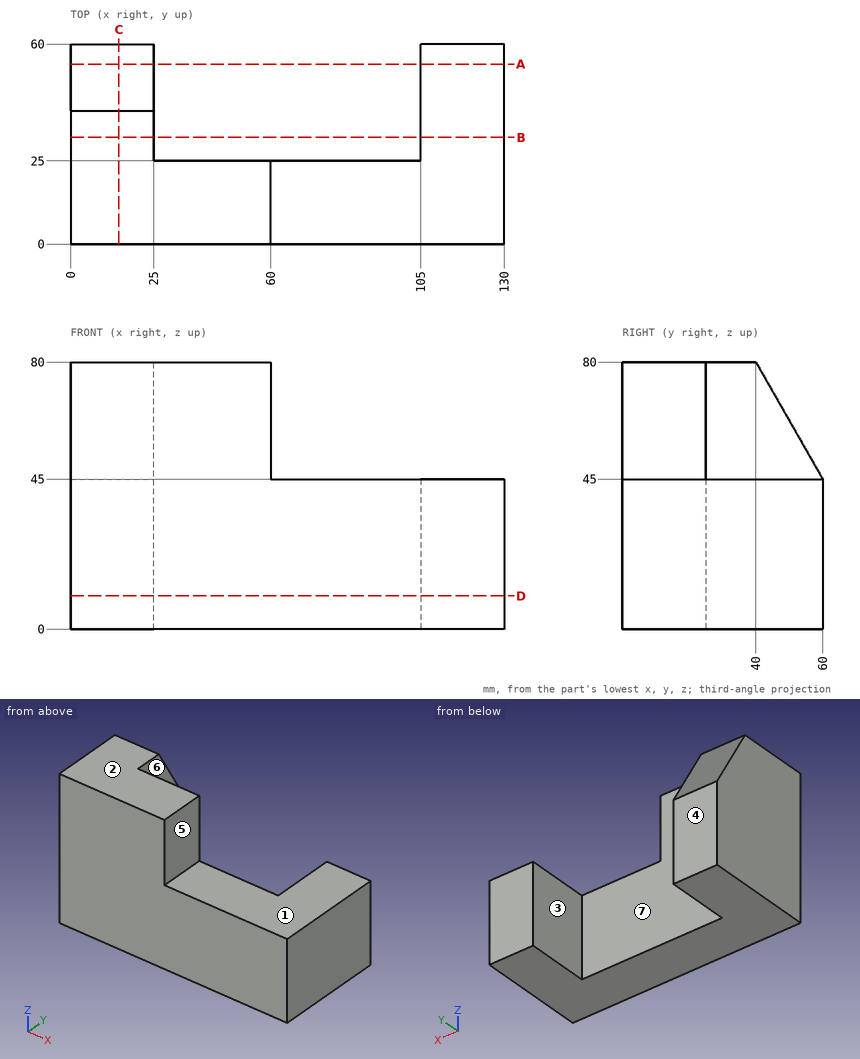
Could you check a few things on this drawing? It's one solid part, dimensions in mm from its lowest x, y, z. A direction names the side the tool comes from. Round coordinates to 2 decimals unless told otherwise and drop trailing zeros. Order: outer loops, then holes, each group sorted by start corner. A loop starts at its lowest first (then second) coordinate and runs counter-clockwise, first axis right, second up. Notation, with made-up numbers: M -3.75,-9.5 L 32.25,-9.5 A15 ccw 32.25,6.5 Z; hole C 47.25,52.5 d3. An arc over 180 degrees is marked long. Use a Markdown table: item, result.
1) Imagine slicing it at B-B (y = 32). List the corners of the cut face in (x, z) for me, then the cut area to 4 significant figures.
Geometry says:
| item | result |
|---|---|
| outline | M 0,0 L 25,0 L 25,80 L 0,80 Z; M 105,0 L 130,0 L 130,45 L 105,45 Z |
| area | 3,125 mm² |
2) I'm going to push flat-ended pins straight in: P1, Ø10.5, axis at y = 51, z = 12.5, coming from the -X side; P2, Ø5, axis at x = 69, z = 40, coming from the +Y side. Where does each tip first touch, or does it pass through?
Geometry says:
| item | result |
|---|---|
| P1 | stops at x = 0 |
| P2 | stops at y = 25 |
3) Imagine slicing it at A-A (y = 54). List the corners of the cut face in (x, z) for me.
Geometry says:
| item | result |
|---|---|
| outline | M 0,0 L 25,0 L 25,55.5 L 0,55.5 Z; M 105,0 L 130,0 L 130,45 L 105,45 Z |
4) Imagine slicing it at D-D (z = 10). List the corners of the cut face in (x, y) for me.
Geometry says:
| item | result |
|---|---|
| outline | M 0,0 L 130,0 L 130,60 L 105,60 L 105,25 L 25,25 L 25,60 L 0,60 Z |
5) Imagine slicing it at C-C (x = 14.5). List the corners of the cut face in (y, z) for me, then the cut area to 3 significant figures.
Geometry says:
| item | result |
|---|---|
| outline | M 0,0 L 60,0 L 60,45 L 40,80 L 0,80 Z |
| area | 4,450 mm² |
6) On a 3-axis mill with a long thin cutter (end or side, diameter ignored), from which of +Z, -Z, +X, -X, +Y, -Y can I reach the whole of each face in a straight line? I mean the marked faces 1, 2 and 3. Say none if no direction works.
Geometry says:
| item | result |
|---|---|
| face 1 | +Z, +X, +Y, -Y |
| face 2 | +Z, +X, -X, +Y, -Y |
| face 3 | +Z, -Z, +Y |
7) If we mould it in two halves opening along X, with no side actions, what happens to the marked faces 4, 5, 6 and 7? For each: +X half, -X half, draft (parallel to the pull), parting line (faces both ways), or undercut.
Geometry says:
| item | result |
|---|---|
| face 4 | draft |
| face 5 | +X half |
| face 6 | undercut |
| face 7 | undercut |
8) If I drill on line 1 along X through (y, z) = (30, 29); line 2 along X through (y, z) = (48, 56.5), over which ranges is the centre line in solid material (lowest first)?
Geometry says:
| item | result |
|---|---|
| line 1 | x = 0 to 25, 105 to 130 |
| line 2 | x = 0 to 25 |
